```python
from build123d import *

# Parameters (mm, degrees)
SKETCH1_R           = 52.07
SKETCH1_R_2         = 9.5123
EXTRUDE1_DEPTH      = 6.35
BOSS_EXTRUDE1_DEPTH = 12.7
CHAMFER3_SIZE       = 0.79502


with BuildPart() as part:
    # Sketch1 → Extrude1 (new, symmetric)
    with BuildSketch(Plane.XY):
        Circle(SKETCH1_R)
        Circle(SKETCH1_R_2, mode=Mode.SUBTRACT)
    extrude(amount=EXTRUDE1_DEPTH, both=True)

    # Sketch3 → Boss-Extrude1 (add)
    with BuildSketch(Plane(origin=(0, 0, -6.35), x_dir=(-1, 0, 0), z_dir=(0, 0, -1))):
        with BuildLine():
            Line((-6.359543229, 7.0739), (6.359543229, 7.0739))
            ThreePointArc((6.359543229, 7.0739), (0, 9.5123), (-6.359543229, 7.0739))
        make_face()
    extrude(amount=-BOSS_EXTRUDE1_DEPTH)

    # Chamfer3
    chamfer3_edges = [part.edges().sort_by_distance(p)[0] for p in [
        (0, -9.5123, -6.35),
        (0, 7.0739, -6.35),
        (0, 7.0739, 6.35),
        (0, -9.5123, 6.35),
    ]]
    chamfer(chamfer3_edges, length=CHAMFER3_SIZE)


solid = part.part
```
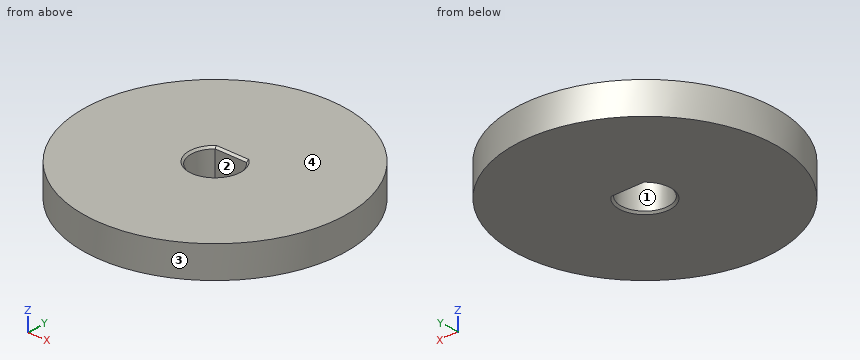
Geometry: final body of the model. Coordinates: model frame, mm. Face numbers are marked on the shaded views. Coordinates: 2 decimals unless noted, no trailing zeros. Order: outer loops, then holes, each group sorted by start corner. A loop starts at its lowest first (then second) coordinate and runs counter-clockwise, first axis right, second up. Notation, with made-up numbers: (48.25, -15) -> (76.25, -15) arc R14 cw to (76.25, 7) -> close; hole circle Ø9 at (72, 79.25). An arc over 180 degrees is marked (long way). Answer in a Markdown table with one row per item.
Item 1: Section B-B on x = 0. Output: boundary loops of the cut face in (y, z), plus the area to 3 significant figures.
Return value:
| item | result |
|---|---|
| outline | (-52.07, -6.35) -> (-10.31, -6.35) -> (-9.51, -5.55) -> (-9.51, 5.55) -> (-10.31, 6.35) -> (-52.07, 6.35) -> close; (7.07, -5.55) -> (7.87, -6.35) -> (52.07, -6.35) -> (52.07, 6.35) -> (7.87, 6.35) -> (7.07, 5.55) -> close |
| area | 1,110 mm² |
Item 2: Section C-C on z = 1.5. Output: boundary loops of the cut face in (x, y), plus the area to 3 significant figures.
Return value:
| item | result |
|---|---|
| outline | circle Ø104.14 at (0, 0); hole (-6.36, 7.07) arc R9.51 ccw (long way) to (6.36, 7.07) -> close |
| area | 8,250 mm² |
Item 3: Ray query, L1, parallel to Y at x = 0, z = 3.5; L2, parallel to X at y = -5, z = -2.25; L3, parallel to X at y = -6.5, z = -1.25. Return the intervals inside material, ascending.
Return value:
| item | result |
|---|---|
| L1 | y = -52.07 to -9.51, 7.07 to 52.07 |
| L2 | x = -51.83 to -8.09, 8.09 to 51.83 |
| L3 | x = -51.66 to -6.95, 6.95 to 51.66 |
Item 4: Section D-D on y = 22. Output: boundary loops of the cut face in (x, z), plus the area to 3 significant figures.
Return value:
| item | result |
|---|---|
| outline | (-47.19, -6.35) -> (47.19, -6.35) -> (47.19, 6.35) -> (-47.19, 6.35) -> close |
| area | 1,200 mm² |
Item 5: Section A-A on y = 0. Output: boundary loops of the cut face in (x, z), plus the area to 3 significant figures.
Return value:
| item | result |
|---|---|
| outline | (-52.07, -6.35) -> (-10.31, -6.35) -> (-9.51, -5.55) -> (-9.51, 5.55) -> (-10.31, 6.35) -> (-52.07, 6.35) -> close; (9.51, -5.55) -> (10.31, -6.35) -> (52.07, -6.35) -> (52.07, 6.35) -> (10.31, 6.35) -> (9.51, 5.55) -> close |
| area | 1,080 mm² |
Item 6: Draft query along Y for the marked faces 1, 2, 3 and 4. Return one class per face: released by +Y, released by -Y, zero draft, split by the parting line, or undercut.
Return value:
| item | result |
|---|---|
| face 1 | undercut |
| face 2 | undercut |
| face 3 | split by the parting line |
| face 4 | zero draft |
Item 7: Contact query for flat-ended pins moving along their axis: P1, Ø1, axis at x = 18.5, z = 2, coming from the -Y side; P2, Ø4, axis at y = -25, z = -3.5, coming from the +X side; P3, Ø3.5, axis at x = 1.5, z = 2.5, coming from the -Y side. Output: stop coordinate, or through.
Return value:
| item | result |
|---|---|
| P1 | stops at y = -48.86 |
| P2 | stops at x = 46.71 |
| P3 | stops at y = -52.07 |
